Design review of the part built by this model. Coordinates are the model's own, in mm. Face numbers are marked on the shaded views. A direction names the side the tool comes from. Give positions to 0.01 mm unless a question says otherwise; leave off trailing zeros. Write each loop counter-clockwise with the first axis right and the second up, starting at its lowest first coordinate (ties: lowest second). Pieces come first, ordered by that corner, then holes. Notation, with made-up numbers: (17.5, 60) - (24.5, 60) arc R20 cw to (24.5, 80) - close; hole circle Ø5 at (-35, 4.5). An arc over 180 degrees is marked (long way). Use a Markdown table: item, result. Add a question column.
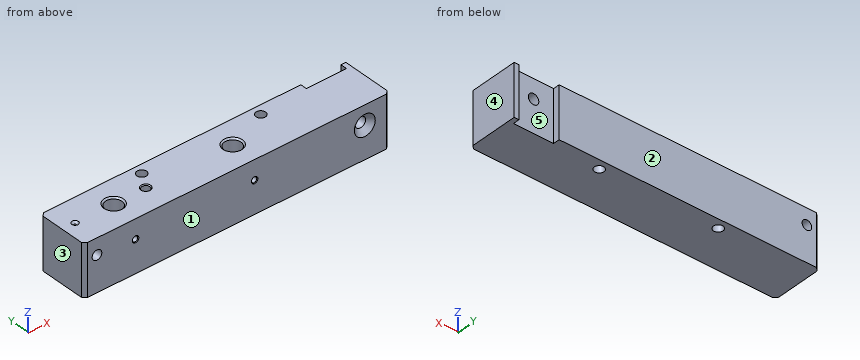
```python
from build123d import *

# Parameters (mm, degrees)
BOSS_EXTRUDE1_DEPTH                                  = 16
M12_TAPPED_HOLE2_D                                   = 10.2
M12_TAPPED_HOLE2_DEPTH                               = 24
M12_TAPPED_HOLE2_CSINK_D                             = 12.05
M12_TAPPED_HOLE2_CSINK_ANGLE                         = 90
M12_TAPPED_HOLE2_TIP                                 = 3.064389157
M4_TAPPED_HOLE1_D                                    = 3.3
M4_TAPPED_HOLE1_DEPTH                                = 11.5
M4_TAPPED_HOLE1_CSINK_D                              = 4.05
M4_TAPPED_HOLE1_CSINK_ANGLE                          = 90
M4_TAPPED_HOLE1_TIP                                  = 0.991420021
SKETCH15_R                                           = 3
CUT_EXTRUDE1_DEPTH                                   = 102.513545894
CSK_FOR_M4_COUNTERSUNK_FLAT_HEAD_SCREW1_D            = 1.5
CSK_FOR_M4_COUNTERSUNK_FLAT_HEAD_SCREW1_DEPTH        = 10
CSK_FOR_M4_COUNTERSUNK_FLAT_HEAD_SCREW1_CSINK_D      = 4
CSK_FOR_M4_COUNTERSUNK_FLAT_HEAD_SCREW1_CSINK_ANGLE  = 90
CSK_FOR_M4_COUNTERSUNK_FLAT_HEAD_SCREW1_TIP          = 0.450645464
M6_TAPPED_HOLE1_D                                    = 5
M6_TAPPED_HOLE1_DEPTH                                = 16
M6_TAPPED_HOLE1_CSINK_D                              = 6.05
M6_TAPPED_HOLE1_CSINK_ANGLE                          = 90
M6_TAPPED_HOLE1_TIP                                  = 1.502151548
SKETCH22_R                                           = 3
CUT_EXTRUDE2_DEPTH                                   = 102.51354591
CSK_FOR_M10_COUNTERSUNK_FLAT_HEAD_SCREW2_D           = 6.5
CSK_FOR_M10_COUNTERSUNK_FLAT_HEAD_SCREW2_DEPTH       = 32
CSK_FOR_M10_COUNTERSUNK_FLAT_HEAD_SCREW2_CSINK_D     = 13
CSK_FOR_M10_COUNTERSUNK_FLAT_HEAD_SCREW2_CSINK_ANGLE = 90
CSK_FOR_M10_COUNTERSUNK_FLAT_HEAD_SCREW2_TIP         = 1.952797012


with BuildPart() as part:
    # Sketch1 → Boss-Extrude1 (new, symmetric)
    with BuildSketch(Plane.XY):
        Polygon((67, 12), (92, 12), (92, 16), (95, 16), (95, -14), (93, -16), (-93, -16), (-95, -14), (-95, 14), (-93, 16), (67, 16), align=None)
    extrude(amount=BOSS_EXTRUDE1_DEPTH, both=True)

    # M12 Tapped Hole2
    with Locations(Plane.XY.offset(16)):
        with Locations((-63, 0), (11, 0)):
            CounterSinkHole(M12_TAPPED_HOLE2_D / 2, M12_TAPPED_HOLE2_CSINK_D / 2, depth=M12_TAPPED_HOLE2_DEPTH, counter_sink_angle=M12_TAPPED_HOLE2_CSINK_ANGLE)
            with Locations((0, 0, -(M12_TAPPED_HOLE2_DEPTH + M12_TAPPED_HOLE2_TIP / 2))):  # 118° drill point
                Cone(0, M12_TAPPED_HOLE2_D / 2, M12_TAPPED_HOLE2_TIP, mode=Mode.SUBTRACT)

    # M4 Tapped Hole1
    with Locations(Plane(origin=(0, -16, 0), x_dir=(-1, 0, 0), z_dir=(0, -1, 0))):
        with Locations((-11, -4), (63, -4)):
            CounterSinkHole(M4_TAPPED_HOLE1_D / 2, M4_TAPPED_HOLE1_CSINK_D / 2, depth=M4_TAPPED_HOLE1_DEPTH, counter_sink_angle=M4_TAPPED_HOLE1_CSINK_ANGLE)
            with Locations((0, 0, -(M4_TAPPED_HOLE1_DEPTH + M4_TAPPED_HOLE1_TIP / 2))):  # 118° drill point
                Cone(0, M4_TAPPED_HOLE1_D / 2, M4_TAPPED_HOLE1_TIP, mode=Mode.SUBTRACT)

    # Sketch15 → Cut-Extrude1 (cut, through all)
    with BuildSketch(Plane.XZ.offset(16)):
        with Locations(Location((-87, 6, 0), (0, 0, 270))):
            Circle(SKETCH15_R)
    extrude(amount=-CUT_EXTRUDE1_DEPTH, mode=Mode.SUBTRACT)

    # CSK for M4 Countersunk Flat Head Screw1
    with Locations(Plane.XY.offset(16)):
        with Locations((-87, 0)):
            CounterSinkHole(CSK_FOR_M4_COUNTERSUNK_FLAT_HEAD_SCREW1_D / 2, CSK_FOR_M4_COUNTERSUNK_FLAT_HEAD_SCREW1_CSINK_D / 2, depth=CSK_FOR_M4_COUNTERSUNK_FLAT_HEAD_SCREW1_DEPTH, counter_sink_angle=CSK_FOR_M4_COUNTERSUNK_FLAT_HEAD_SCREW1_CSINK_ANGLE)
            with Locations((0, 0, -(CSK_FOR_M4_COUNTERSUNK_FLAT_HEAD_SCREW1_DEPTH + CSK_FOR_M4_COUNTERSUNK_FLAT_HEAD_SCREW1_TIP / 2))):  # 118° drill point
                Cone(0, CSK_FOR_M4_COUNTERSUNK_FLAT_HEAD_SCREW1_D / 2, CSK_FOR_M4_COUNTERSUNK_FLAT_HEAD_SCREW1_TIP, mode=Mode.SUBTRACT)

    # M6 Tapped Hole1
    with Locations(Plane.XY.offset(16)):
        with Locations((-43, 0)):
            CounterSinkHole(M6_TAPPED_HOLE1_D / 2, M6_TAPPED_HOLE1_CSINK_D / 2, depth=M6_TAPPED_HOLE1_DEPTH, counter_sink_angle=M6_TAPPED_HOLE1_CSINK_ANGLE)
            with Locations((0, 0, -(M6_TAPPED_HOLE1_DEPTH + M6_TAPPED_HOLE1_TIP / 2))):  # 118° drill point
                Cone(0, M6_TAPPED_HOLE1_D / 2, M6_TAPPED_HOLE1_TIP, mode=Mode.SUBTRACT)

    # Sketch22 → Cut-Extrude2 (cut, through all)
    with BuildSketch(Plane.XY.offset(16)):
        with Locations((-37, 10)):
            Circle(SKETCH22_R)
        with Locations((37, 10)):
            Circle(SKETCH22_R)
    extrude(amount=-CUT_EXTRUDE2_DEPTH, mode=Mode.SUBTRACT)

    # CSK for M10 Countersunk Flat Head Screw2
    with Locations(Plane(origin=(0, -16, 0), x_dir=(-1, 0, 0), z_dir=(0, -1, 0))):
        with Locations((-79.5, -4)):
            CounterSinkHole(CSK_FOR_M10_COUNTERSUNK_FLAT_HEAD_SCREW2_D / 2, CSK_FOR_M10_COUNTERSUNK_FLAT_HEAD_SCREW2_CSINK_D / 2, depth=CSK_FOR_M10_COUNTERSUNK_FLAT_HEAD_SCREW2_DEPTH, counter_sink_angle=CSK_FOR_M10_COUNTERSUNK_FLAT_HEAD_SCREW2_CSINK_ANGLE)
            with Locations((0, 0, -(CSK_FOR_M10_COUNTERSUNK_FLAT_HEAD_SCREW2_DEPTH + CSK_FOR_M10_COUNTERSUNK_FLAT_HEAD_SCREW2_TIP / 2))):  # 118° drill point
                Cone(0, CSK_FOR_M10_COUNTERSUNK_FLAT_HEAD_SCREW2_D / 2, CSK_FOR_M10_COUNTERSUNK_FLAT_HEAD_SCREW2_TIP, mode=Mode.SUBTRACT)


solid = part.part
```
(1) Mouldability with a two-part tool opening along Y and no side actions: class the marked faces 1, 2 and 3 as +Y half, -Y half, draft (parallel to the pull), parting line (faces both ways), or undercut.
(2) Add section B-B (x = 37). State the section outline as (y, z) points, and give its area (3 significant figures).
(3) For line 1 along X through (y, z) = (0, 11); line 2 along Z through (x, y) = (-87, 8); line 3 along X through (y, z) = (9, 14.5), list the stretches that pass through material, from the lowest coordinate up.
(4) Tool access review of the marked faces 4 and 5: name each direction out of +Z, -Z, +X, -X, +Y, -Y from which nothing blocks a thin tool from reaching the whole face with its end or side.
(5) Add section A-A (x = 79.5). State the section outline as (y, z) points.
(6) Insertion check: pin 1 (12.5 mm diameter, centred on x = 78, z = 6, fed in from +Y); pin 2 (1.2 mm diameter, centred on x = -87, y = 0, fed in from +Z); pin 3 (2 mm diameter, centred on x = -63, z = 4, fed in from -Y). Each pin has a flat end and moves straight along its axis. Give the tip position at first contact, or say it passes through.
Answers follow:
| question | item | result |
|---|---|---|
| 1 | face 1 | -Y half |
| 1 | face 2 | +Y half |
| 1 | face 3 | draft |
| 2 | outline | (-16, -16) - (7, -16) - (7, 16) - (-16, 16) - close; (13, -16) - (16, -16) - (16, 16) - (13, 16) - close |
| 2 | area | 832 mm^2 |
| 3 | line 1 | -95 to -87.75, -86.25 to -68.1, -57.9 to -45.5, -40.5 to 5.9, 16.1 to 95 |
| 3 | line 2 | -16 to 3, 9 to 16 |
| 3 | line 3 | -95 to -39.83, -34.17 to 34.17, 39.83 to 95 |
| 4 | face 4 | +Z, -Z, +X, +Y, -Y |
| 4 | face 5 | +Z, -Z, +Y |
| 5 | outline | (-16, -16) - (12, -16) - (12, 0.75) - (-12.75, 0.75) - (-16, -2.5) - close; (-16, 10.5) - (-12.75, 7.25) - (12, 7.25) - (12, 16) - (-16, 16) - close |
| 6 | pin 1 | y = 12 |
| 6 | pin 2 | z = 3.06 |
| 6 | pin 3 | y = 5 |
